Autodesk Inventor part; units mm, degrees
ref_plane "YZ Plane" through (0, 0, 0) normal (1, 0, 0) x (0, 1, 0)
ref_plane "XZ Plane" through (0, 0, 0) normal (0, 1, 0) x (-1, 0, 0)
ref_plane "XY Plane" through (0, 0, 0) normal (0, 0, 1) x (1, 0, 0)
sketch "Sketch1" plane through (0, 0, 0) normal (0, 0, 1) x (1, 0, 0)
  line L0 (0, 0) -> (0, 137.0131)
  line L1 (-11.7886, 12.2907) -> (-39.6863, 18.4755) construction
  line L2 (-39.6863, 18.4755) -> (-33.3297, 47.1481) construction
  line L3 (-33.3297, 47.1481) -> (-5.432, 40.9633) construction
  line L4 (-5.432, 40.9633) -> (-11.7886, 12.2907) construction
  line L5 (-39.6863, 18.4755) -> (-5.432, 40.9633) construction
  line L6 (-33.3297, 47.1481) -> (-11.7886, 12.2907) construction
  circle A0 centre (-53.975, 12.7) radius 3.175
  circle A1 centre (-53.975, 12.7) radius 9.525
  line L7 (0, 0) -> (-54.5315, 3.1913) construction
  line L8 (-62.4238, 17.0982) -> (0, 137.0131) construction
  line L9 (-27.1302, 45.7737) -> (-37.4529, 28.5497) construction
  line L10 (-11.6315, 42.3377) -> (-9.5552, 22.3649) construction
  line L11 (-19.3809, 44.0557) -> (-25.7374, 15.3831) construction
  line L12 (0, 104.775) -> (-15.0457, 108.1106) construction
  line L13 (-35.3766, 8.5768) -> (-19.8779, 5.1408) construction
  line L14 (-19.8779, 5.1408) -> (-21.2523, -1.0586) construction
  line L15 (-21.2523, -1.0586) -> (-36.751, 2.3773) construction
  line L16 (-36.751, 2.3773) -> (-35.3766, 8.5768) construction
  line L17 (-35.3766, 8.5768) -> (-44.7305, 2.6177) construction
  line L18 (-19.8779, 5.1408) -> (-17.2457, 1.0092) construction
  line L19 (-5.432, 40.9633) -> (-33.3297, 47.1481) construction
  line L20 (-33.3297, 47.1481) -> (-32.2475, 52.0296) construction
  line L21 (-32.2475, 52.0296) -> (-4.3498, 45.8448) construction
  line L22 (-4.3498, 45.8448) -> (-5.432, 40.9633) construction
  line L23 (-53.2878, 15.7997) -> (-53.975, 12.7) construction
  line L24 (-53.975, 12.7) -> (-57.0747, 13.3872) construction
  line L25 (-27.6272, 6.8588) -> (-34.4992, -24.1386) construction
  line L26 (-31.8676, 50.076) -> (-5.5198, 44.2349) construction
  line L27 (-5.5198, 44.2349) -> (-4.489, 48.8845) construction
  line L28 (-4.489, 48.8845) -> (-30.8368, 54.7256) construction
  line L29 (-30.8368, 54.7256) -> (-31.8676, 50.076) construction
  line L30 (-31.3522, 52.4008) -> (-5.0044, 46.5597) construction
  circle A2 centre (-29.0274, 51.8854) radius 1.4732 construction
  circle A3 centre (-22.8279, 50.5111) radius 1.4732 construction
  circle A4 centre (-16.6284, 49.1367) radius 1.4732
  circle A5 centre (-10.4289, 47.7623) radius 1.4732
  circle A6 centre (-7.6985, 96.7513) radius 1.4732
  line L31 (-53.975, 12.7) -> (-5.4185, 105.9762) construction
  line L32 (-31.2085, 56.4341) -> (0, 49.5153) construction
  circle A7 centre (-7.6985, 96.7513) radius 4.7625 construction
  line L33 (-4.7625, 48.9451) -> (-4.7625, 105.8308)
  line L34 (-26.3948, 55.3669) -> (-7.323, 92.0036) construction
  line L35 (-3.5958, 94.3328) -> (-4.7625, 94.5914) construction
  line L36 (-17.2457, 1.0092) -> (0, 1.0092) construction
  line L37 (0, 1.0092) -> (0, -2.1658) construction
  line L38 (0, -2.1658) -> (-17.2457, -2.1658) construction
  line L39 (-17.2457, -2.1658) -> (-17.2457, 1.0092) construction
  circle A8 centre (-12.7, 7.9375) radius 1.5875 construction
  line L40 (-12.7, 7.9375) -> (0, 7.9375) construction
  line L41 (0, 7.9375) -> (-17.2457, 1.0092)
  circle A9 centre (-12.7, 7.9375) radius 3.175 construction
  line L42 (-9.525, 7.9375) -> (-9.525, 4.111) construction
  line L43 (-9.525, 7.9375) -> (0, 7.9375) construction
  line L44 (-17.9187, 46.9837) -> (-16.8879, 51.6333) construction
  line L45 (-12.4942, 45.7811) -> (-26.2381, -16.2137) construction
  line L46 (0, 53.6985) -> (0, 7.9375) construction
  line L47 (-26.2381, -16.2137) -> (-20.0386, -17.5881) construction
  line L48 (-20.0386, -17.5881) -> (-8.7313, 7.9375)
  circle A10 centre (-12.7, 6.35) radius 1.4224
  line L49 (0, 13.4938) -> (-4.7625, 13.4938) construction
  line L50 (-4.7625, 13.4938) -> (-4.7625, 24.6063) construction
  line L51 (-4.7625, 24.6063) -> (0, 24.6063) construction
  line L52 (0, 24.6063) -> (0, 13.4938) construction
  line L53 (-4.7625, 19.05) -> (0, 19.05) construction
  circle A11 centre (-2.3813, 19.05) radius 1.4224
  line L54 (-20.7405, 8.5842) -> (-9.7454, 58.18) construction
  line L55 (-9.7454, 58.18) -> (-3.5459, 56.8056) construction
  line L56 (-3.5459, 56.8056) -> (-14.5411, 7.2098) construction
  line L57 (-14.5411, 7.2098) -> (-20.7405, 8.5842) construction
  line L58 (-12.7, 6.35) -> (-12.7, 7.9375) construction
  line L59 (-11.5442, 1.5875) -> (-9.525, 1.5875) construction
  line L60 (-9.525, 1.5875) -> (-9.525, 7.9375) construction
  line L61 (-9.525, 7.9375) -> (-11.5442, 7.9375) construction
  line L62 (-11.5442, 7.9375) -> (-11.5442, 1.5875) construction
  line L63 (-9.7454, 58.18) -> (-15.9449, 59.5544) construction
  line L64 (-18.8691, 53.6985) -> (0, 53.6985) construction
  line L65 (-9.7454, 58.18) -> (-17.3193, 53.3549) construction
  arc A12 (-10.2313, 55.9882) -> (-11.9373, 58.6659) centre (-11.0843, 57.3271) ccw construction
  line L66 (-4.7625, 57.15) -> (0, 57.15) construction
  circle A13 centre (-2.3813, 57.15) radius 1.4224
  circle A14 centre (-2.3813, 63.5) radius 1.4224
  line L67 (0, 7.9375) -> (-45.2378, 7.9375) construction
  line L68 (-45.2378, 7.9375) -> (-45.2378, -28.575) construction
  line L69 (-45.2378, -28.575) -> (0, -28.575)
  line L70 (0, -28.575) -> (0, 7.9375)
  line L71 (-45.2378, -28.575) -> (-62.6076, 8.6746)
  line L72 (-60.0032, 20.0747) -> (-18.8691, 53.6985) construction
  line L73 (-20.0386, -17.5881) -> (-20.0386, -28.575) construction
  line L74 (-20.2435, 47.4991) -> (-19.2127, 52.1487) construction
  line L75 (-12.7, -28.575) -> (-12.7, -1.0217)
  circle A15 centre (-23.8125, -19.05) radius 1.7526
  circle A16 centre (-15.875, -14.2875) radius 1.7526
  circle A17 centre (-23.8125, -19.05) radius 3.175 construction
  circle A18 centre (-2.3813, 69.85) radius 1.4224
  circle A19 centre (-2.3813, 76.2) radius 1.4224
  circle A20 centre (-15.875, -14.2875) radius 3.175 construction
  circle A21 centre (-46.0375, -19.05) radius 1.7526
  arc A22 (0, 104.775) -> (-15.0457, 108.1106) centre (-7.9697, 104.427) ccw construction
  circle A23 centre (-7.9697, 104.427) radius 1.4224
  line L76 (-7.9697, 104.427) -> (-15.0457, 108.1106) construction
  line L77 (-7.9697, 104.427) -> (0, 104.775) construction
  line L78 (0, 43.0112) -> (-20.2435, 47.4991)
  line L79 (-20.2435, 47.4991) -> (-25.4, 94.1319)
  line L80 (-25.4, 94.1319) -> (3.175, 135.4256)
  line L81 (0, 122.468) -> (-20.4707, 92.8859)
  line L82 (-20.4707, 92.8859) -> (-15.8846, 51.4108)
  line L83 (-15.8846, 51.4108) -> (0, 47.8893)
  line L84 (-20.4707, 92.8859) -> (-4.7625, 91.7678)
  line L85 (3.175, 135.4256) -> (3.175, 47.8893)
  line L86 (3.175, 47.8893) -> (0, 47.8893)
  line L87 (-25.4, 94.1319) -> (-4.7625, 48.9451)
  line L88 (-19.9433, 93.648) -> (-4.7625, 60.4089)
  point P0 (-22.5591, 29.7194)
  point P1 (-20.7484, 1.2142)
  point P2 (-36.3367, 4.2458)
  point P3 (-49.5768, 21.1488)
  point P4 (-11.1125, 7.9375)
  point P5 (-11.4283, 6.9872)
  point P6 (-11.9574, 7.9375)
  point P7 (-13.9717, 6.9872)
  point P8 (-9.525, 6.1457)
  point P9 (-10.6215, 3.6705)
  point P10 (0, 130.8374)
  point P11 (-19.5658, 92.8214)
  dimension "d74" = 6.35
  dimension "d14" = 29.3687
  dimension "d15" = 28.575
  dimension "d16" = 12.5
  dimension "d17" = 6.35
  dimension "d19" = 53.975
  dimension "d22" = 19.05
  dimension "d23" = 7.9375
  dimension "d24" = 19.05
  dimension "d26" = 102.5
  dimension "d29" = 6.35
  dimension "d31" = 7.9375
  dimension "d34" = 5
  dimension "d35" = 26.9875
  dimension "d38" = 31.75
  dimension "d40" = 26.9875
  dimension "d41" = 4.7625
  dimension "d42" = 2.9464
  dimension "d43" = 2.3813
  dimension "d46" = 6.35
  dimension "d51" = 2.9464
  dimension "d52" = 92.075
  dimension "d53" = 6.35
  dimension "d54" = 9.525
  dimension "d55" = 4.7625
  dimension "d56" = 4.7625
  dimension "d60" = 12.7
  dimension "d61" = 3.175
  dimension "d63" = 3.175
  dimension "d66" = 3.175
  dimension "d67" = 12.7
  dimension "d72" = 8.7312
  dimension "d73" = 7.9375
  dimension "d80" = 12.7
  dimension "d82" = 7.9375
  dimension "d83" = 63.5
  dimension "d85" = 6.35
  dimension "d86" = 104.775
  dimension "d87" = 2.8448
  dimension "d88" = 4.7625
  dimension "d89" = 11.1125
  dimension "d90" = 2.8448
  dimension "d91" = 19.05
  dimension "d92" = 6.35
  dimension "d93" = 50.8
  dimension "d94" = 25.4
  dimension "d95" = 8.7312
  dimension "d96" = 9.525
  dimension "d97" = 6.35
  dimension "d99" = 6.35
  dimension "d101" = 3.175
  dimension "d106" = 2.8448
  dimension "d107" = 57.15
  dimension "d110" = 6.35
  dimension "d136" = 3.175
  dimension "d138" = 28.575
  dimension "d139" = 12.7
  dimension "d140" = 3.5052
  dimension "d141" = 3.5052
  dimension "d142" = 9.525
  dimension "d143" = 3.175
  dimension "d144" = 11.1125
  dimension "d145" = 6.35
  dimension "d146" = 14.2875
  dimension "d149" = 6.35
extrude "Extrusion1" add sketch "Sketch1" along normal blind 4.7625 contours L83 L33 L84 L88 L81 L0 | L0 L80 L85 L86 | L81 L82 L87 L80 L0 | L87 L82 L84 L88 L33 | L88 L84 L81
fillet "Fillet7" radius 4.7625 5 edges at (-4.7625, 91.7678, 2.3813) (-25.4, 94.1319, 2.3813) (-4.7625, 48.9451, 2.3813) (0, 47.8893, 2.3813) (3.175, 47.8893, 2.3813)
fillet "Fillet8" radius 2.3813 2 edges at (-19.5658, 92.8214, 2.3813) (-4.7625, 60.4089, 2.3813)
equation "\"d56\" = d55"
properties part number "Uprights" material "Steel, Alloy"
For this review, take the finished solid that the model builds, in its own axes (mm). A direction names the side the tool comes from. Round coordinates to 2 decimals unless told otherwise and drop trailing zeros. Order: outer loops, then holes, each group sorted by start corner. A loop starts at its lowest first (then second) coordinate and runs counter-clockwise, first axis right, second up. Notation, with made-up numbers: M -20,-1.5 L -13,-1.5 A19 cw -13,32.5 Z; hole C 86,72 d8. An arc over 180 degrees is marked long. Use a Markdown table: item, result. Add a question column.
Item 1: Add section B-B, the plane x = -10.75. Give the boundary of the cut face in (y, z).
Item 2: Add section C-C, the plane z = 3.4. State how many separate pieces and enclosed holes the cut face has, then the cut area to 3 significant figures.
Item 3: Add section A-A, the plane y = 83. Give the boundary of the cut face in (x, z) (1 decimal), then the cut area to 3 significant figures.
Item 4: Add section D-D, the plane x = -20.25. Give the boundary of the cut face in (y, z).
Item 5: Mouldability with a two-part tool opening along X and no side actions: class faces 3 (the flat face through (-12.42, 92.313, 2.348)), 4 (the cylindrical face through (-24.684, 94.103, 2.415)), 5 (the flat face through (3.175, 95, 2)) as released by +X, released by -X, zero draft, split by the parting line, or undercut.
Item 6: Tool access review of faces 1 (the flat face through (-4.762, 79, 2)), 2 (the flat face through (-8, 93, 0)): name each direction out of +Z, -Z, +X, -X, +Y, -Y from which nothing blocks a thin tool from reaching the whole face with its end or side.
Item 7: To check wall thickness, follow line 1 along Y through (x, z) = (-1.25, 2.6); line 2 along Y through (x, z) = (-8.25, 2.65); line 3 along X through (y, z) = (76.5, 0.35) (1 decimal). State the ranges of each line that lie inside material, in increasing order.
Item 8: Insertion check: pin 1 (1 mm diameter, centred on x = -8, z = 1.5, fed in from +Y); pin 2 (2 mm diameter, centred on x = -5.5, z = 2.5, fed in from -Y). Each pin has a flat end and moves straight along its axis. Give the tip position at first contact, or say it passes through.
Geometry results:
| question | item | result |
|---|---|---|
| 1 | outline | M 62.06,0 L 73.52,0 L 73.52,4.76 L 62.06,4.76 Z; M 92.19,0 L 115.3,0 L 115.3,4.76 L 92.19,4.76 Z |
| 2 | separate pieces | 1 |
| 2 | enclosed holes | 7 |
| 2 | area | 1,160 mm² |
| 3 | outline | M -20.3,0 L -15.1,0 L -15.1,4.8 L -20.3,4.8 Z; M -4.8,0 L 3.2,0 L 3.2,4.8 L -4.8,4.8 Z |
| 3 | area | 62.7 mm² |
| 4 | outline | M 82.86,0 L 101.57,0 L 101.57,4.76 L 82.86,4.76 Z |
| 5 | face 3 | undercut |
| 5 | face 4 | released by -X |
| 5 | face 5 | released by +X |
| 6 | face 1 | +Z, -Z |
| 6 | face 2 | -Z, +X, -X, +Y, -Y |
| 7 | line 1 | y = 48.7 to 56.29, 58.01 to 62.64, 64.36 to 68.99, 70.71 to 75.34, 77.06 to 129.03 |
| 7 | line 2 | y = 56.58 to 69.25, 91.92 to 95.39, 98.12 to 103.03, 105.82 to 118.92 |
| 7 | line 3 | x = -17.3 to -12.1, -4.8 to -3.8, -1 to 3.2 |
| 8 | pin 1 | stops at y = 120 |
| 8 | pin 2 | stops at y = 49.69 |
